from build123d import *

# Parameters (mm, degrees)
BOSS_EXTRUDE1_DEPTH = 49.27
SKETCH12_W          = 2.099999999999998
SKETCH12_H          = 6.83
SKETCH12_W_2        = 2.0999999999999996
SKETCH12_H_2        = 6.829999999999998
SKETCH12_W_3        = 2.1000000000000014
BOSS_EXTRUDE2_DEPTH = 1.57
SKETCH4_R           = 4.91
CUT_EXTRUDE3_DEPTH  = 22
SKETCH5_R           = 2
CUT_EXTRUDE4_DEPTH  = 5
SKETCH7_R           = 1.5
CUT_EXTRUDE5_DEPTH  = 34.41594267711148
FILLET4_R           = 3
FILLET5_R           = 3
SKETCH13_R          = 1.6049999999999995
SKETCH13_R_2        = 1.6049999999999962
SKETCH13_R_3        = 1.605
CUT_EXTRUDE6_DEPTH  = 2


with BuildPart() as part:
    # Sketch2 → Boss-Extrude1 (new body)
    with BuildSketch(Plane(origin=(0, 0, 0), x_dir=(1, 0, 0), z_dir=(0, 1, 0))):
        Polygon((-15.325000000000001, 12.36), (15.324999999999998, 12.36), (15.325, -12.360000000000003), (-15.324999999999996, -12.360000000000003), align=None)
    extrude(amount=BOSS_EXTRUDE1_DEPTH)

    # Sketch12 → Boss-Extrude2 (add)
    with BuildSketch(Plane.XZ):
        with Locations((-14.274999999999997, 8.945000000000004)):
            Rectangle(SKETCH12_W, SKETCH12_H)
        with Locations((-14.275000000000002, -8.944999999999999)):
            Rectangle(SKETCH12_W_2, SKETCH12_H_2)
        with Locations((14.274999999999999, 8.945000000000004)):
            Rectangle(SKETCH12_W_3, SKETCH12_H)
        with Locations((14.274999999999999, -8.944999999999999)):
            Rectangle(SKETCH12_W_3, SKETCH12_H_2)
    extrude(amount=BOSS_EXTRUDE2_DEPTH)

    # Sketch4 → Cut-Extrude3 (cut)
    with BuildSketch(Plane(origin=(0, 49.27, 0), x_dir=(1, 0, 0), z_dir=(0, 1, 0))):
        with Locations(Location((0, 0, 0), (0, 0, 270))):
            Circle(SKETCH4_R)
    extrude(amount=-CUT_EXTRUDE3_DEPTH, mode=Mode.SUBTRACT)

    # Sketch5 → Cut-Extrude4 (cut)
    with BuildSketch(Plane(origin=(0, 27.270000000000003, 0), x_dir=(1, 0, 0), z_dir=(0, 1, 0))):
        with Locations(Location((0, 0, 0), (0, 0, 270))):
            Circle(SKETCH5_R)
    extrude(amount=-CUT_EXTRUDE4_DEPTH, mode=Mode.SUBTRACT)

    # Sketch7 → Cut-Extrude5 (cut, through all)
    with BuildSketch(Plane(origin=(0, 22.270000000000003, 0), x_dir=(1, 0, 0), z_dir=(0, 1, 0))):
        with Locations(Location((0, 0, 0), (0, 0, 270))):
            Circle(SKETCH7_R)
    extrude(amount=-CUT_EXTRUDE5_DEPTH, mode=Mode.SUBTRACT)

    # Fillet4
    # the kernel refuses this fillet: 3 mm, written as the material it takes off along each edge
    with BuildSketch(Plane(origin=(0, 27.270000000000003, 0), x_dir=(-1.8e-16, 0, 1), z_dir=(-1, 0, -1.8e-16))) as fillet4_piece_1:
        with BuildLine():
            CenterArc((5, -2.9986496961132367), FILLET4_R, 91.7191313208778, 88.2808686791222)
            Line((2, -2.9986496961132367), (1.94, -2.9986496961132367))
            Line((1.94, -2.9986496961132367), (1.94, 0))
            Line((1.94, 0), (2, 0.05999999999999872))
            ThreePointArc((2, 0.05999999999999872), (3.455, 0.05999999999999872), (4.9082, 0.05997299392226552))
            Line((4.9082, 0.05997299392226552), (4.91, 0))
        make_face()
    revolve(axis=Axis((0, 27.270000000000003, 0), (0, 1, 0)), mode=Mode.SUBTRACT)

    # Fillet5
    # the kernel refuses this fillet: 3 mm, written as the material it takes off along each edge
    with BuildSketch(Plane(origin=(0, 22.270000000000003, 0), x_dir=(-1.8e-16, 0, 1), z_dir=(-1, 0, -1.8e-16))) as fillet5_piece_1:
        with BuildLine():
            CenterArc((4.5, -1.6583123951831418), FILLET5_R, 146.44269023799268, 33.55730976200732)
            Line((2.0000000000025064, -1.66267e-12), (1.9500000000025566, 0.03316624790196698))
            ThreePointArc((1.9500000000025566, 0.03316624790196698), (1.7500000000012532, 0.05999999999999872), (1.5, 0.05999999999999872))
            Line((1.5, 0.05999999999999872), (1.44, 0))
            Line((1.44, 0), (1.44, -1.6583123951831418))
            Line((1.44, -1.6583123951831418), (1.5, -1.6583123951831418))
        make_face()
    revolve(axis=Axis((0, 22.270000000000003, 0), (0, 1, 0)), mode=Mode.SUBTRACT)

    # Sketch13 → Cut-Extrude6 (cut)
    with BuildSketch(Plane(origin=(15.324999999999998, 0, -1.08e-15), x_dir=(-7e-17, 0, -1), z_dir=(1, 0, -7e-17))):
        with Locations((-8.630000000000006, 42.27)):
            Circle(SKETCH13_R)
        with Locations((8.629999999999999, 42.27)):
            Circle(SKETCH13_R_2)
        with Locations((-8.630000000000006, 6.870000000000001)):
            Circle(SKETCH13_R_3)
        with Locations((8.629999999999999, 6.870000000000001)):
            Circle(SKETCH13_R_3)
    extrude(amount=-CUT_EXTRUDE6_DEPTH, mode=Mode.SUBTRACT)


solid = part.part
The listing builds one solid part. Answer for the finished solid, in the listing's coordinates (mm). A direction names the side the tool comes from. Give positions to 0.01 mm unless a question says otherwise; leave off trailing zeros. Loops run counter-clockwise (first coordinate to the right, second up) from the corner with the lowest first, then second, coordinate; pieces in that order, holes last. Notation, with made-up numbers: (-16, 14) - (0, 14) arc R17 cw to (0, 38) - close; hole circle Ø4 at (27.25, -36). An arc over 180 degrees is marked (long way). Use one line per item in the form item = value.
1. The mould has two halves that part along Z. Classify faces 1 (the face through (0, 24, 12.36)), 2 (the face through (-2, 23, 0)), 3 (the face through (-13.225, -1, 9)): pulls with the +Z half, pulls with the -Z half, needs draft (parallel to the pull), parting line crosses it, or undercut.
Calculated:
face_1 = pulls with the +Z half
face_2 = undercut
face_3 = needs draft
2. Section B-B on y = 42.27 is taken. Give the vertices of the cut face in (x, z) (3 decimals), then the cut area to 3 significant figures.
Calculated:
outline = (-15.325, -12.36) - (15.325, -12.36) - (15.325, -10.235) - (13.325, -10.235) - (13.325, -7.025) - (15.325, -7.025) - (15.325, 7.025) - (13.325, 7.025) - (13.325, 10.235) - (15.325, 10.235) - (15.325, 12.36) - (-15.325, 12.36) - close; hole circle Ø9.82 at (0, 0)
area = 669 mm^2
3. Given pin 1 Ø1.5 at (x, z) = (4, -3.5) entering from -Y, flat-ended and moving along its own axis, determine where the tip first touches the part or whether it passes through.
Calculated:
pin_1 = 0
4. Which of the six approach directions +Z, -Z, +X, -X, +Y, -Y give full straight-line access (tool end or side, diameter ignored) to faces 4 (the face through (-14, -1, -5.53)), 5 (the face through (13.225, -1, 9)), 6 (the face through (14.34, 8.46, -8.42)), 7 (the face through (-4.793, 38.424, -1.064))?
Calculated:
face_4 = +X, -X, -Y
face_5 = +Z, -Z, -Y
face_6 = +X
face_7 = +Y
5. Section A-A on x = 0 is taken. Give the vertices of the cut face in (y, z).
Calculated:
outline = (0, -12.36) - (49.27, -12.36) - (49.27, -4.91) - (27.27, -4.91) arc R3 ccw to (24.27, -2) - (22.27, -2) arc R3 ccw to (20.61, -1.5) - (0, -1.5) - close; (0, 1.5) - (20.61, 1.5) arc R3 ccw to (22.27, 2) - (24.27, 2) arc R3 ccw to (27.27, 4.91) - (49.27, 4.91) - (49.27, 12.36) - (0, 12.36) - close
6. Section D-D on x = 8 is taken. Give the vertices of the cut face in (y, z), then the cut area to 3 significant figures.
Calculated:
outline = (0, -12.36) - (49.27, -12.36) - (49.27, 12.36) - (0, 12.36) - close
area = 1,220 mm^2
7. Section C-C on z = 10.75 is taken. Give the vertices of the cut face in (x, y) (3 decimals).
Calculated:
outline = (-15.325, -1.57) - (-13.225, -1.57) - (-13.225, 0) - (13.225, 0) - (13.225, -1.57) - (15.325, -1.57) - (15.325, 49.27) - (-15.325, 49.27) - close
8. Find the intervals of material crossed by line 1 along Y through (x, z) = (14.55, 8.63) (3 decimals); line 2 along X through (y, z) = (35.25, 0) (3 decimals); line 3 along Y through (x, z) = (1, -6.5), in increasing order. Write a range as [from, to].
Calculated:
line_1 = [-1.57, 5.265], [8.475, 40.665], [43.875, 49.27]
line_2 = [-15.325, -4.91], [4.91, 15.325]
line_3 = [0, 49.27]
